Here's how the part is built. I have some questions about the finished solid (model axes, mm). Give positions to 0.01 mm unless a question says otherwise; leave off trailing zeros. Order: outer loops, then holes, each group sorted by start corner. A loop starts at its lowest first (then second) coordinate and runs counter-clockwise, first axis right, second up. Notation, with made-up numbers: M 10,-16.75 L 30,-16.75 A21 cw 30,8.25 Z; hole C -24.75,78 d8. An arc over 180 degrees is marked long. Use CSV: the item, a comma, the result in double quotes. Start each with the question number.
```python
from build123d import *

# Parameters (mm, degrees)
SKETCH2_W           = 160
SKETCH2_H           = 15
BOSS_EXTRUDE1_DEPTH = 6
BOSS_EXTRUDE2_DEPTH = 6
SKETCH5_R           = 1.5
CUT_EXTRUDE1_DEPTH  = 82.352627493
CUT_EXTRUDE2_DEPTH  = 82.352627493
FILLET1_R           = 7


with BuildPart() as part:
    # Sketch2 → Boss-Extrude1 (new body)
    with BuildSketch(Plane(origin=(0, 0, 0), x_dir=(1, 0, 0), z_dir=(0, 1, 0))):
        Rectangle(SKETCH2_W, SKETCH2_H)
    extrude(amount=BOSS_EXTRUDE1_DEPTH)

    # Sketch4 → Boss-Extrude2 (add)
    with BuildSketch(Plane(origin=(0, 0, 0), x_dir=(1, 0, 0), z_dir=(0, 1, 0))):
        with BuildLine():
            Line((-45, -7.5), (-33, -7.5))
            ThreePointArc((-33, -7.5), (-39, -13.5), (-45, -7.5))
        make_face()
    extrude(amount=BOSS_EXTRUDE2_DEPTH)

    # Sketch5 → Cut-Extrude1 (cut, through all)
    with BuildSketch(Plane(origin=(0, 6, 0), x_dir=(1, 0, 0), z_dir=(0, 1, 0))):
        with Locations(Location((-77, 0, 0), (0, 0, 270))):
            Circle(SKETCH5_R)
        with Locations(Location((-39, -9.5, 0), (0, 0, 270))):
            Circle(SKETCH5_R)
        with Locations(Location((77, -4.5, 0), (0, 0, 270))):
            Circle(SKETCH5_R)
    extrude(amount=-CUT_EXTRUDE1_DEPTH, mode=Mode.SUBTRACT)

    # Sketch6 → Cut-Extrude2 (cut, through all)
    with BuildSketch(Plane(origin=(0, 6, 0), x_dir=(1, 0, 0), z_dir=(0, 1, 0))):
        Polygon((80, 0), (80, 7.5), (30, 7.5), align=None)
    extrude(amount=-CUT_EXTRUDE2_DEPTH, mode=Mode.SUBTRACT)

    # Fillet1
    fillet1_edges = [part.edges().sort_by_distance(p)[0] for p in [
        (-80, 3, -7.5),
        (-80, 3, 7.5),
    ]]
    fillet(fillet1_edges, radius=FILLET1_R)


solid = part.part
```
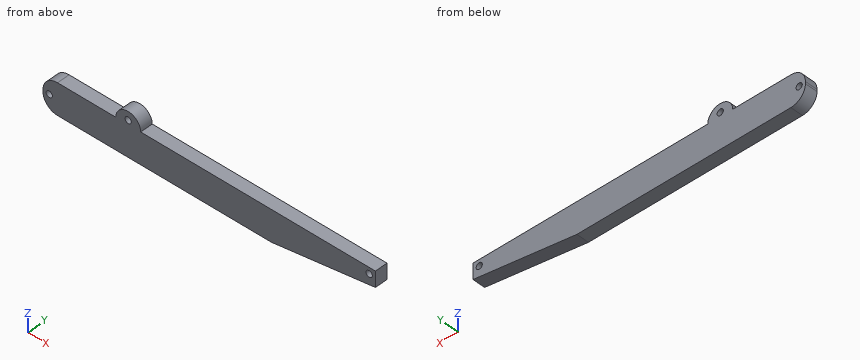
Q1. I need wall thicknesses on line 1 (Z direction, x = 13, y = 1.9); line 2 (X direction, y = 1.5, z = 4.5); line 3 (Z direction, x = -77, y = 3.9). Which ranges of each line are inside material? Lowest first, please. Write a range as [from, to].
Q2. Imagine slicing it at C-C, the plane z = 4.5. Please give me the cut outline in (x, y).
Q3. Imagine slicing it at A-A, the plane x = 77. Please give me the cut outline in (y, z).
Q4. Imagine slicing it at B-B, the plane y = 3.9. Please give me the cut outline in (x, z).
Q5. For P1, Ø2.5, axis at x = -39, z = 9.5, coming from the +Y side, with a flat end and sliding along its axis, tell me the tip position at first contact or that it passes through.
Q6. Imagine slicing it at D-D, the plane x = 16. Please give me the cut outline in (y, z).
Reply:
1,line 1,"z = [-7.5, 7.5]"
1,line 2,"x = [-78.74, 75.5], [78.5, 80]"
1,line 3,"z = [-6.24, -1.5], [1.5, 6.24]"
2,outline,"M -78.74,0 L 75.5,0 L 75.5,6 L -78.74,6 Z; M 78.5,0 L 80,0 L 80,6 L 78.5,6 Z"
3,outline,"M 0,-0.45 L 6,-0.45 L 6,3 L 0,3 Z; M 0,6 L 6,6 L 6,7.5 L 0,7.5 Z"
4,outline,"M -80,-0.5 A7 ccw -73,-7.5 L 30,-7.5 L 80,0 L 80,7.5 L -33,7.5 A6 ccw -45,7.5 L -73,7.5 A7 ccw -80,0.5 Z; hole C -77,0 d3; hole C -39,9.5 d3; hole C 77,4.5 d3"
5,P1,"passes through"
6,outline,"M 0,-7.5 L 6,-7.5 L 6,7.5 L 0,7.5 Z"
